Source: CAD feature listing. Evaluate the final solid. Frame: model axes, mm. A direction names the side the tool comes from. Give positions to 0.01 mm unless a question says otherwise; leave off trailing zeros. Loops run counter-clockwise (first coordinate to the right, second up) from the corner with the lowest first, then second, coordinate; pieces in that order, holes last. Notation, with made-up numbers: (45.25, -10) -> (84.25, -10) arc R27 ccw to (84.25, 13) -> close; hole circle Ø9 at (84, 25.5). An arc over 180 degrees is marked (long way). Put each result on its own line as item: value.
```python
from build123d import *

# Parameters (mm, degrees)
SKETCH1_W           = 64
SKETCH1_H           = 16
BOSS_EXTRUDE1_DEPTH = 5
SKETCH2_W           = 30
SKETCH2_H           = 16
BOSS_EXTRUDE2_DEPTH = 55
SKETCH3_R           = 7
CUT_EXTRUDE1_DEPTH  = 55


with BuildPart() as part:
    # Sketch1 → Boss-Extrude1 (new body)
    with BuildSketch(Plane(origin=(0, 0, 0), x_dir=(1, 0, 0), z_dir=(0, 1, 0))):
        Rectangle(SKETCH1_W, SKETCH1_H)
    extrude(amount=BOSS_EXTRUDE1_DEPTH)

    # Sketch2 → Boss-Extrude2 (add)
    with BuildSketch(Plane(origin=(0, 5, 0), x_dir=(1, 0, 0), z_dir=(0, 1, 0))):
        Rectangle(SKETCH2_W, SKETCH2_H)
    extrude(amount=BOSS_EXTRUDE2_DEPTH)

    # Sketch3 → Cut-Extrude1 (cut)
    with BuildSketch(Plane.XY.offset(8)):
        with Locations((0, 40)):
            Circle(SKETCH3_R)
    extrude(amount=-CUT_EXTRUDE1_DEPTH, mode=Mode.SUBTRACT)


solid = part.part
```
(1) Section C-C on z = -2. Return loops of the section in (x, y).
Calculated:
outline: (-32, 0) -> (32, 0) -> (32, 5) -> (15, 5) -> (15, 60) -> (-15, 60) -> (-15, 5) -> (-32, 5) -> close; hole circle Ø14 at (0, 40)
(2) Reachability of faces 4 (the flat face through (0, 30, 8)), 5 (the flat face through (15, 32, 0)), 6 (the flat face through (-24, 5, 0)) from +Z, -Z, +X, -X, +Y, -Y: full face, straight path, thin tool, end or side. Return the list, or none.
Calculated:
face 4: +Z, +X, -X, +Y, -Y
face 5: +Z, -Z, +X, +Y
face 6: +Z, -Z, -X, +Y
(3) Section A-A on y = 40. Return loops of the section in (x, z), then the cut area to 3 significant figures.
Calculated:
outline: (-15, -8) -> (-7, -8) -> (-7, 8) -> (-15, 8) -> close; (7, -8) -> (15, -8) -> (15, 8) -> (7, 8) -> close
area: 256 mm²
(4) Section B-B on x = 0. Return loops of the section in (y, z).
Calculated:
outline: (0, -8) -> (33, -8) -> (33, 8) -> (0, 8) -> close; (47, -8) -> (60, -8) -> (60, 8) -> (47, 8) -> close
(5) Line query: probe 1 along Y at (x, z) = (0, -1); probe 2 along Y at (x, z) = (-22.5, -3.5); probe 3 along X at (y, z) = (43, 0.5). Output: solid intervals per line, ascending. Write a range as from..to.
Calculated:
probe 1: y = 0..33, 47..60
probe 2: y = 0..5
probe 3: x = -15..-6.32, 6.32..15
(6) First-contact query: P1, Ø3, axis at y = 16.5, z = -2, coming from the +X side; P2, Ø8, axis at y = 37.5, z = -3, coming from the -X side. Flat tips, straight axial feed; report the tip coordinate or a pass-through.
Calculated:
P1: stops at x = 15
P2: stops at x = -15
(7) Section D-D on y = 51.5. Return loops of the section in (x, z).
Calculated:
outline: (-15, -8) -> (15, -8) -> (15, 8) -> (-15, 8) -> close
(8) Draft query along X for faces 1 (the cylindrical face through (-0.91, 46.94, 0.11)), 2 (the flat face through (32, 2, 0)), 3 (the flat face through (-32, 2, 0)). Return one class per face: released by +X, released by -X, zero draft, split by the parting line, or undercut.
Calculated:
face 1: undercut
face 2: released by +X
face 3: released by -X
